Verification items for the finished model (mm, model axes). Face numbers are marked on the shaded views. Coordinates: 2 decimals unless noted, no trailing zeros. Write each loop counter-clockwise with the first axis right and the second up, starting at its lowest first coordinate (ties: lowest second). Pieces come first, ordered by that corner, then holes. Notation, with made-up numbers: M 36.25,-37 L 94.25,-37 A4 cw 94.25,-31 Z; hole C 22.25,72 d5. An arc over 180 degrees is marked long. One line per item, written item: value.
```python
from build123d import *

# Parameters (mm, degrees)
SKIZZE1_R                       = 4
SKIZZE1_R_2                     = 3
AUFSATZ_LINEAR_AUSTRAGEN1_DEPTH = 14.25
FASE1_SIZE                      = 0.2


with BuildPart() as part:
    # Skizze1 → Aufsatz-Linear austragen1 (new body)
    with BuildSketch(Plane(origin=(0, 0, 0), x_dir=(1, 0, 0), z_dir=(0, 1, 0))):
        with Locations(Location((0, 0, 0), (0, 0, 90))):
            Circle(SKIZZE1_R)
        with Locations(Location((0, 0, 0), (0, 0, 90))):
            Circle(SKIZZE1_R_2, mode=Mode.SUBTRACT)
    extrude(amount=AUFSATZ_LINEAR_AUSTRAGEN1_DEPTH)

    # Fase1
    fase1_edges = [part.edges().sort_by_distance(p)[0] for p in [
        (0, 0, 4),
        (0, 14.25, 4),
        (0, 0, 3),
        (0, 14.25, 3),
    ]]
    chamfer(fase1_edges, length=FASE1_SIZE)


solid = part.part
```
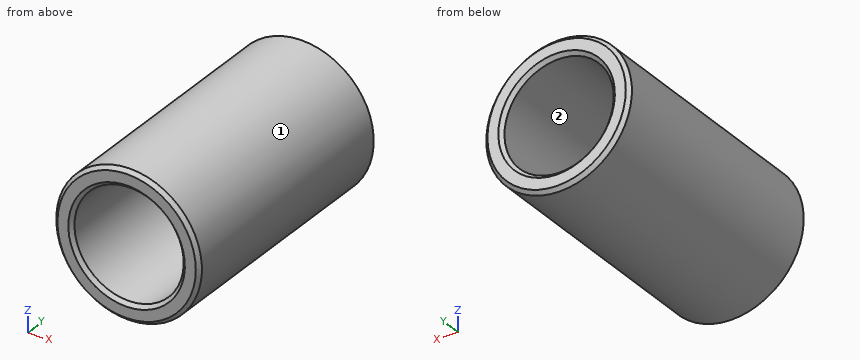
Item 1: Cross-section at A-A, the plane z = 0. Enter the section's corners in (x, y).
The answers:
outline: M -4,0.2 L -3.8,0 L -3.2,0 L -3,0.2 L -3,14.05 L -3.2,14.25 L -3.8,14.25 L -4,14.05 Z; M 3,0.2 L 3.2,0 L 3.8,0 L 4,0.2 L 4,14.05 L 3.8,14.25 L 3.2,14.25 L 3,14.05 Z
Item 2: Scan lines: line 1 (X direction, y = 9, z = 0); line 2 (X direction, y = 9.75, z = 2.75). Record each from-to range of solid material in increasing order.
The answers:
line 1: x = -4 to -3, 3 to 4
line 2: x = -2.9 to -1.2, 1.2 to 2.9
Item 3: Cross-section at C-C, the plane y = 10.75. Enter the section's corners in (x, z).
The answers:
outline: C 0,0 d8; hole C 0,0 d6
Item 4: Draft check along Z on the marked faces 1 and 2. Enter one of: released by +Z, released by -Z, zero draft, split by the parting line, or undercut.
The answers:
face 1: split by the parting line
face 2: undercut
Item 5: Go/stop test with flat-tipped pins: P1, Ø1.5, axis at x = -3, y = 12.5, coming from the +Z side; P2, Ø1, axis at x = -2, y = 2.5, coming from the -Z side; P3, Ø1, axis at y = 8, z = -2, coming from the +X side. Record where each tip stops, or that it passes through.
The answers:
P1: stops at z = 3.31
P2: stops at z = -3.71
P3: stops at x = 3.71
Item 6: Cross-section at B-B, the plane x = 0. Enter the section's corners in (y, z), and give its area (3 significant figures).
The answers:
outline: M 0,-3.8 L 0.2,-4 L 14.05,-4 L 14.25,-3.8 L 14.25,-3.2 L 14.05,-3 L 0.2,-3 L 0,-3.2 Z; M 0,3.2 L 0.2,3 L 14.05,3 L 14.25,3.2 L 14.25,3.8 L 14.05,4 L 0.2,4 L 0,3.8 Z
area: 28.3 mm²
